Input: dimensioned drawing with shaded views. Units: mm. Origin: part minimum x, y, z. Coordinates: 2 decimals unless noted, no trailing zeros. Write each loop counter-clockwise with the first axis right and the second up, starting at its lowest first coordinate (ties: lowest second). Pieces come first, ordered by that corner, then holes. Notation, with made-up numbers: (85, 71.5) - (142, 71.5) arc R24 cw to (142, 85.5) - close; hole circle Ø9 at (57.25, -4). An arc over 180 degrees is marked (long way). One line per question, with ' | ' between items.
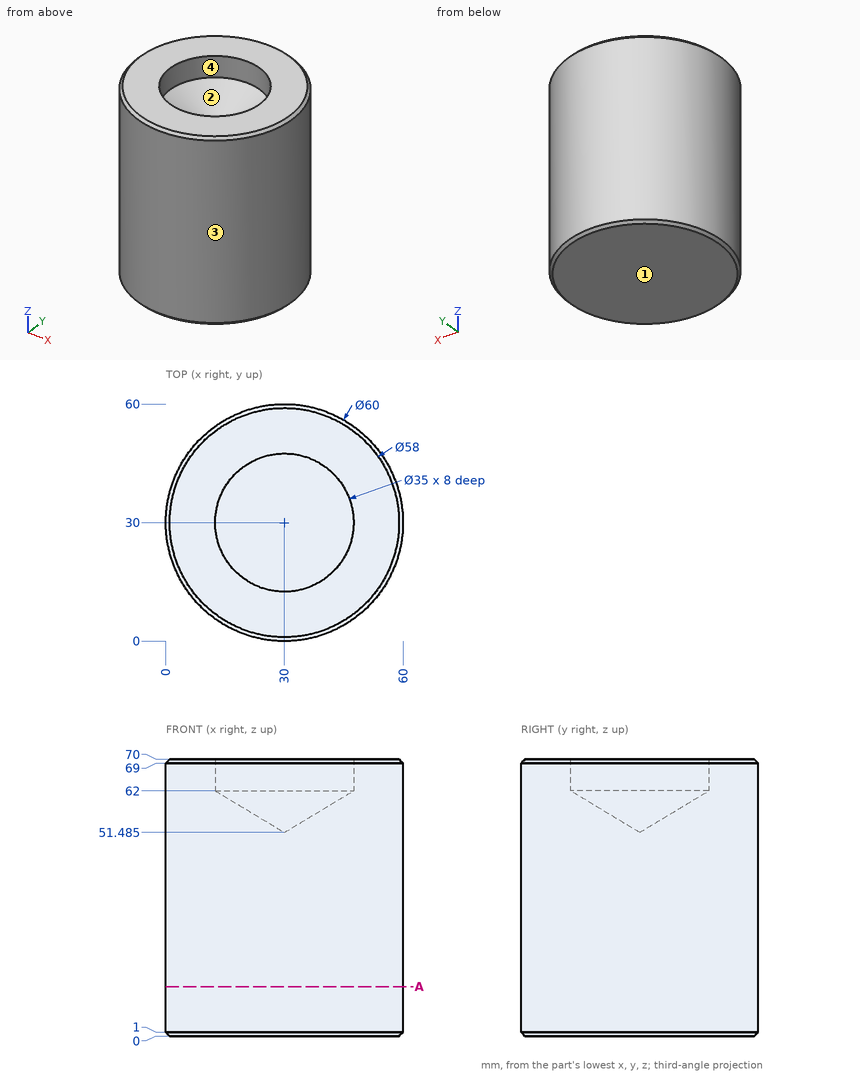
Item 1: Cut plane A-A on z = 12.5. Return loops of the section in (x, y).
Check sheet entries:
outline: circle Ø60 at (30, 30)
Item 2: Pin query (flat end, axial travel): pin 1 Ø1.5 at (x, y) = (48.5, 53) entering from -Z; pin 2 Ø5 at (x, y) = (23.5, 22) entering from +Z; pin 3 Ø5 at (x, z) = (17, 9.5) entering from +Y; pin 4 Ø2 at (x, z) = (37, 43.5) entering from +Y. Return the tip coordinate at first contact, or that it passes through.
Check sheet entries:
pin 1: z = 0 | pin 2: z = 59.18 | pin 3: y = 58.1 | pin 4: y = 59.39
Item 3: Mould query, pull axis Y, two halves, no side actions, for the marked faces 1, 2, 3 and 4. Classes: pulls with the +Y half, pulls with the -Y half, needs draft (parallel to the pull), parting line crosses it, or undercut.
Check sheet entries:
face 1: needs draft | face 2: undercut | face 3: parting line crosses it | face 4: undercut
Item 4: Ray query, line 1 along Y through (x, z) = (30, 65.75); line 2 along X through (y, z) = (31, 16.5); line 3 along Y through (x, z) = (16, 6). Return the intervals inside material, ascending. Write a range as [from, to].
Check sheet entries:
line 1: [0, 12.5], [47.5, 60] | line 2: [0.02, 59.98] | line 3: [3.47, 56.53]
